Build history of the part. All positions in model axes, mm. A direction names the side the tool comes from. Give positions to 0.01 mm unless a question says otherwise; leave off trailing zeros. Loops run counter-clockwise (first coordinate to the right, second up) from the corner with the lowest first, then second, coordinate; pieces in that order, holes last. Notation, with made-up numbers: (-2, 6) -> (18, 6) arc R15 cw to (18, 29) -> close; hole circle Ø7 at (-4.5, 62). An arc over 180 degrees is marked (long way). Answer as a JSON object with one key per item and string values. Group by question number.
from build123d import *

# Parameters (mm, degrees)
SKETCH1_R           = 3.45
SKETCH1_R_2         = 1.65
BOSS_EXTRUDE1_DEPTH = 5
SKETCH2_W           = 11
SKETCH2_H           = 15
BOSS_EXTRUDE2_DEPTH = 3
FILLET1_R           = 2
CUT_EXTRUDE1_DEPTH  = 22.499883744
FILLET2_R           = 8


with BuildPart() as part:
    # Sketch1 → Boss-Extrude1 (new body)
    with BuildSketch(Plane.XY):
        Circle(SKETCH1_R)
        Circle(SKETCH1_R_2, mode=Mode.SUBTRACT)
    extrude(amount=BOSS_EXTRUDE1_DEPTH)

    # Sketch2 → Boss-Extrude2 (add)
    with BuildSketch(Plane(origin=(0, 0, 0), x_dir=(-1, 0, 0), z_dir=(0, 0, -1))):
        with Locations((-7.15, -9.15)):
            Rectangle(SKETCH2_W, SKETCH2_H)
    extrude(amount=-BOSS_EXTRUDE2_DEPTH)

    # Fillet1
    # the kernel refuses this fillet: 2 mm, written as the material it adds along each edge
    with BuildSketch(Plane(origin=(0, 0, 3), x_dir=(0.5811301681486029, 0.8138106215008357, 0), z_dir=(-0.8138106215008357, 0.5811301681486029, 0))) as fillet1_piece_1_section:
        with BuildLine():
            CenterArc((3.45 + FILLET1_R, -FILLET1_R), FILLET1_R, 90, 90)
            Line((3.45 + FILLET1_R, 0), (3.45 + FILLET1_R, FILLET1_R * 0.02))
            Line((3.45 + FILLET1_R, FILLET1_R * 0.02), (3.45 - FILLET1_R * 0.02, FILLET1_R * 0.02))
            Line((3.45 - FILLET1_R * 0.02, FILLET1_R * 0.02), (3.45 - FILLET1_R * 0.02, -FILLET1_R))
            Line((3.45 - FILLET1_R * 0.02, -FILLET1_R), (3.45, -FILLET1_R))
        make_face()
    fillet1_piece_1 = revolve(axis=Axis((0, 0, 3), (0, 0, -1)), revolution_arc=198.93985607, mode=Mode.PRIVATE)
    fillet1_piece_1 = split(fillet1_piece_1, bisect_by=Plane(origin=(1.65, -2.775668714, 3.387031985), z_dir=(1, 0, 0)), keep=Keep.TOP, mode=Mode.PRIVATE)
    fillet1_piece_1 = split(fillet1_piece_1, bisect_by=Plane(origin=(2.775669412, -1.65, 3.387031985), z_dir=(0, -1, 0)), keep=Keep.TOP, mode=Mode.PRIVATE)
    add(fillet1_piece_1)
    with BuildSketch(Plane(origin=(1.65, -3.029851482, 3), x_dir=(-0.9765037028672113, -0.21550062247386903, 0), z_dir=(0, 0, -1))) as fillet1_piece_2:
        with BuildLine():
            CenterArc((2.472126505, -1.921296938), FILLET1_R, 106.126978769, 86.317920605)
            Line((0.519119099, -2.352298183), (0.480058951, -2.360918208))
            Line((0.480058951, -2.360918208), (-0.039060148, -0.008620025))
            Line((-0.039060148, -0.008620025), (0.011110681, 0.038425939))
            ThreePointArc((0.011110681, 0.038425939), (0.958296229, -0.095762782), (1.905481778, 0.038425939))
            Line((1.905481778, 0.038425939), (1.916592459, 0))
        make_face()
    extrude(amount=3)
    with BuildSketch(Plane(origin=(3.029851482, -1.65, 3), x_dir=(0.21550062247386917, 0.9765037028672113, 0), z_dir=(0, 0, -1))) as fillet1_piece_3:
        with BuildLine():
            CenterArc((2.472126505, 1.921296938), FILLET1_R, 167.555100626, 86.317920605)
            Line((0.519119099, 2.352298183), (0.480058951, 2.360918208))
            Line((0.480058951, 2.360918208), (-0.039060148, 0.008620025))
            Line((-0.039060148, 0.008620025), (0.011110681, -0.038425939))
            ThreePointArc((0.011110681, -0.038425939), (0.958296229, 0.095762782), (1.905481778, -0.038425939))
            Line((1.905481778, -0.038425939), (1.916592459, 0))
        make_face()
    extrude(amount=3)
    with BuildSketch(Plane(origin=(0, 0, 3), x_dir=(0.5811301681486029, 0.8138106215008357, 0), z_dir=(-0.8138106215008357, 0.5811301681486029, 0))) as fillet1_piece_4a_section:
        with BuildLine():
            CenterArc((3.45 + FILLET1_R, -FILLET1_R), FILLET1_R, 90, 90)
            Line((3.45 + FILLET1_R, 0), (3.45 + FILLET1_R, FILLET1_R * 0.02))
            Line((3.45 + FILLET1_R, FILLET1_R * 0.02), (3.45 - FILLET1_R * 0.02, FILLET1_R * 0.02))
            Line((3.45 - FILLET1_R * 0.02, FILLET1_R * 0.02), (3.45 - FILLET1_R * 0.02, -FILLET1_R))
            Line((3.45 - FILLET1_R * 0.02, -FILLET1_R), (3.45, -FILLET1_R))
        make_face()
    fillet1_piece_4a = revolve(axis=Axis((0, 0, 3), (0, 0, -1)), revolution_arc=198.93985607, mode=Mode.PRIVATE)
    fillet1_piece_4a = split(fillet1_piece_4a, bisect_by=Plane(origin=(3.505644008, -1.65, 3.43409217), z_dir=(0, 1, 0)), keep=Keep.TOP, mode=Mode.PRIVATE)
    with BuildSketch(Plane(origin=(3.029851482, -1.65, 9.022245937), x_dir=(0.21550062247386909, 0.9765037028672113, 0), z_dir=(0, 0, -1))) as fillet1_piece_4b_section:
        with BuildLine():
            CenterArc((2.472126505, 1.921296938), FILLET1_R, 167.555100626, 86.317920605)
            Line((0.519119099, 2.352298183), (0.480058951, 2.360918208))
            Line((0.480058951, 2.360918208), (-0.039060148, 0.008620025))
            Line((-0.039060148, 0.008620025), (0.011110681, -0.038425939))
            ThreePointArc((0.011110681, -0.038425939), (0.958296229, 0.095762782), (1.905481778, -0.038425939))
            Line((1.905481778, -0.038425939), (1.916592459, 0))
        make_face()
    fillet1_piece_4b = extrude(amount=9.022245937, mode=Mode.PRIVATE)
    fillet1_piece_4b = split(fillet1_piece_4b, bisect_by=Plane(origin=(3.781400642, -1.225418489, 3), z_dir=(0, 0, 1)), keep=Keep.TOP, mode=Mode.PRIVATE)
    fillet1_piece_4 = fillet1_piece_4a & fillet1_piece_4b
    add(fillet1_piece_4)
    with BuildSketch(Plane(origin=(1.65, -3.029851482, 9.022245937), x_dir=(-0.9765037028672113, -0.2155006224738689, 0), z_dir=(0, 0, -1))) as fillet1_piece_5a_section:
        with BuildLine():
            CenterArc((2.472126505, -1.921296938), FILLET1_R, 106.126978769, 86.317920605)
            Line((0.519119099, -2.352298183), (0.480058951, -2.360918208))
            Line((0.480058951, -2.360918208), (-0.039060148, -0.008620025))
            Line((-0.039060148, -0.008620025), (0.011110681, 0.038425939))
            ThreePointArc((0.011110681, 0.038425939), (0.958296229, -0.095762782), (1.905481778, 0.038425939))
            Line((1.905481778, 0.038425939), (1.916592459, 0))
        make_face()
    fillet1_piece_5a = extrude(amount=9.022245937, mode=Mode.PRIVATE)
    fillet1_piece_5a = split(fillet1_piece_5a, bisect_by=Plane(origin=(1.225418489, -3.781400642, 3), z_dir=(0, 0, 1)), keep=Keep.TOP, mode=Mode.PRIVATE)
    with BuildSketch(Plane(origin=(0, 0, 3), x_dir=(0.5811301681486029, 0.8138106215008357, 0), z_dir=(-0.8138106215008357, 0.5811301681486029, 0))) as fillet1_piece_5b_section:
        with BuildLine():
            CenterArc((3.45 + FILLET1_R, -FILLET1_R), FILLET1_R, 90, 90)
            Line((3.45 + FILLET1_R, 0), (3.45 + FILLET1_R, FILLET1_R * 0.02))
            Line((3.45 + FILLET1_R, FILLET1_R * 0.02), (3.45 - FILLET1_R * 0.02, FILLET1_R * 0.02))
            Line((3.45 - FILLET1_R * 0.02, FILLET1_R * 0.02), (3.45 - FILLET1_R * 0.02, -FILLET1_R))
            Line((3.45 - FILLET1_R * 0.02, -FILLET1_R), (3.45, -FILLET1_R))
        make_face()
    fillet1_piece_5b = revolve(axis=Axis((0, 0, 3), (0, 0, -1)), revolution_arc=198.93985607, mode=Mode.PRIVATE)
    fillet1_piece_5b = split(fillet1_piece_5b, bisect_by=Plane(origin=(1.65, -3.505643385, 3.43409212), z_dir=(-1, 0, 0)), keep=Keep.TOP, mode=Mode.PRIVATE)
    fillet1_piece_5 = fillet1_piece_5a & fillet1_piece_5b
    add(fillet1_piece_5)

    # Sketch3 → Cut-Extrude1 (cut, through all)
    with BuildSketch(Plane(origin=(0, 0, 0), x_dir=(-1, 0, 0), z_dir=(0, 0, -1))):
        with BuildLine():
            Line((-4.65, -16.65), (-4.65, -8.65))
            ThreePointArc((-4.65, -8.65), (-3.783315491, -6.452721713), (-1.65, -5.438749856))
            Line((-1.65, -5.438749856), (-1.65, -16.65))
            Line((-1.65, -16.65), (-4.65, -16.65))
        make_face()
    extrude(amount=-CUT_EXTRUDE1_DEPTH, mode=Mode.SUBTRACT)

    # Fillet2
    fillet2_edges = [part.edges().sort_by_distance(p)[0] for p in [
        (1.65, -5.438749856, 1.5),
    ]]
    fillet(fillet2_edges, radius=FILLET2_R)


solid = part.part
(1) Saw through at C-C on z = 3.7. List the corners of the cut face in (x, y).
(2) Saw through at B-B on y = 0. List the corners of the cut face in (x, z), plus the area to 3 significant figures.
(3) Saw through at D-D on x = 7.75. List the corners of the cut face in (y, z).
(4) Saw through at A-A on x = 0. List the corners of the cut face in (y, z), plus the area to 3 significant figures.
(5) Probe line 1 along Y through (x, z) = (5.25, 1.1); line 2 along Y through (x, z) = (0, 3.5); line 3 along X through (y, z) = (-14, 1.95). List the from-to ranges inside material, lowest first. Write a range as [from, to].
(6) 3-axis set-ups, long thin cutter, end or side, ignore diameter. For faces 4 (the flat face through (8, -9, 3)), 5 (the flat face through (4.65, -13, 1)), 6 (the flat face through (7, -7, 0)): which of +Z, -Z, +X, -X, +Y, -Y reach the whole face in a straight line?
(7) Pull direction Y, two halves, no side cores. Call faces 1 (the cylindrical face through (-1.216, 1.115, 2.465)), 2 (the flat face through (9, -1.65, 2)), 3 (the flat face through (0, -2, 5)): pulls with the +Y half, pulls with the -Y half, needs draft (parallel to the pull), parting line crosses it, or undercut.
(8) Pin check, flat tip, straight feed: pin 1 (3 mm diameter, centred on x = 6.5, y = -13, fed in from +Z). Stop position of the tip, or through.
Calculated:
{
 "1": {"outline": "(-0.22, -3.44) arc R2 cw to (0.85, -3.84) arc R3.93 ccw to (3.84, -0.85) arc R2 cw to (3.44, 0.22) arc R3.45 ccw (long way) to start; hole circle Ø3.3 at (0, 0)"},
 "2": {"outline": "(-3.45, 0) -> (-1.65, 0) -> (-1.65, 5) -> (-3.45, 5) -> close; (1.65, 0) -> (3.47, 0) -> (3.47, 4.72) arc R2 cw to (3.45, 5) -> (1.65, 5) -> close", "area": "18.1 mm^2"},
 "3": {"outline": "(-16.65, 0) -> (-1.65, 0) -> (-1.65, 3) -> (-16.65, 3) -> close"},
 "4": {"outline": "(-3.47, 0) -> (-1.65, 0) -> (-1.65, 5) -> (-3.45, 5) arc R2 cw to (-3.47, 4.72) -> close; (1.65, 0) -> (3.45, 0) -> (3.45, 5) -> (1.65, 5) -> close", "area": "18.1 mm^2"},
 "5": {"line 1": "y = [-16.65, -1.64]", "line 2": "y = [-3.47, -1.65], [1.65, 3.45]", "line 3": "x = [4.65, 12.65]"},
 "6": {"face 4": "+Z, +X, -Y", "face 5": "+Z, -Z, -X, -Y", "face 6": "-Z, +X, -X, +Y, -Y"},
 "7": {"face 1": "undercut", "face 2": "pulls with the +Y half", "face 3": "needs draft"},
 "8": {"pin 1": "stops at z = 3"}
}
